For this review, take the finished solid that the model builds, in its own axes (mm). Coordinates: 2 decimals unless noted, no trailing zeros. Write each loop counter-clockwise with the first axis right and the second up, starting at its lowest first coordinate (ties: lowest second). Pieces come first, ordered by that corner, then holes. Notation, with made-up numbers: (-10.5, 54.25) -> (40.5, 54.25) arc R5 ccw to (40.5, 62.25) -> close; hole circle Ø7 at (51, 32). An arc over 180 degrees is marked (long way). One line per item, written item: value. Start each with the question number.
1) For probe 1 along Y at (x, z) = (23.55, -66.4); probe 2 along Y at (x, z) = (0, -67), list the stretches that pass through material, from the lowest coordinate up. Write a range as from..to.
2) Add section B-B (x = 15.75). State the section outline as (y, z) points, and give its area (3 significant figures).
3) Add section D-D (x = 0). State the section outline as (y, z) points.
4) Add section C-C (z = -66.8). State the section outline as (x, y) points, and give its area (3 significant figures).
5) Add section A-A (y = -23.55). State the section outline as (x, z) points, and give its area (3 significant figures).
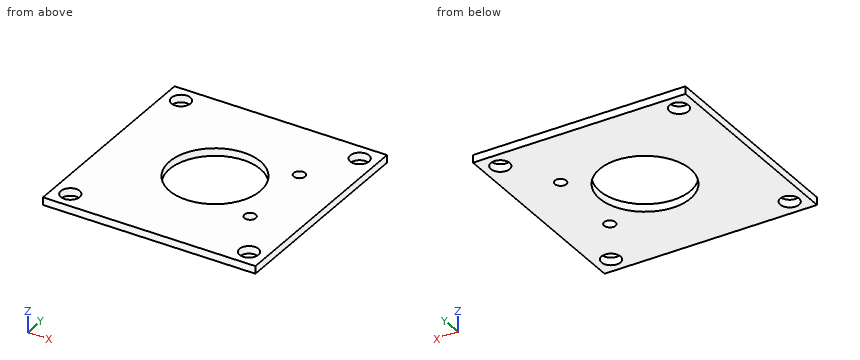
from build123d import *

# Parameters (mm, degrees)
BOX274_W                    = 56
BOX274_H                    = 56
BOX274_DEPTH                = 2
CYLINDER704_R               = 1.5
CYLINDER704_DEPTH           = 20
CYLINDER705_R               = 1.5
CYLINDER705_DEPTH           = 20
COMPOUND417_PLACEMENT_ANGLE = 90
BOX272_W                    = 20
BOX272_H                    = 8
BOX272_DEPTH                = 3
BOX271_W                    = 20
BOX271_H                    = 8
BOX271_DEPTH                = 3
BOX273_W                    = 20
BOX273_H                    = 8
BOX273_DEPTH                = 3
BOX269_W                    = 20
BOX269_H                    = 8
BOX269_DEPTH                = 3
CYLINDER697_R               = 12
CYLINDER697_DEPTH           = 20
CYLINDER702_R               = 5
CYLINDER702_DEPTH           = 4
CYLINDER689_R               = 5
CYLINDER689_DEPTH           = 4
CYLINDER693_R               = 5
CYLINDER693_DEPTH           = 4
CYLINDER698_R               = 5
CYLINDER698_DEPTH           = 4
CYLINDER699_R               = 2.5
CYLINDER699_DEPTH           = 20
CYLINDER690_R               = 2.5
CYLINDER690_DEPTH           = 20
CYLINDER694_R               = 2.5
CYLINDER694_DEPTH           = 20
CYLINDER700_R               = 2.5
CYLINDER700_DEPTH           = 20
CYLINDER696_R               = 3
CYLINDER696_DEPTH           = 5
CYLINDER696_PLACEMENT_ANGLE = 22.5
CYLINDER688_R               = 3
CYLINDER688_DEPTH           = 5
CYLINDER688_PLACEMENT_ANGLE = 67.5
CYLINDER691_R               = 3
CYLINDER691_DEPTH           = 5
CYLINDER691_PLACEMENT_ANGLE = 202.5
CYLINDER692_R               = 3
CYLINDER692_DEPTH           = 5
CYLINDER692_PLACEMENT_ANGLE = 112.5
COMPOUND416_PLACEMENT_ANGLE = 45
CYLINDER703_R               = 1.5
CYLINDER703_DEPTH           = 30
CYLINDER703_PLACEMENT_ANGLE = 22.5
CYLINDER695_R               = 1.5
CYLINDER695_DEPTH           = 30
CYLINDER695_PLACEMENT_ANGLE = 67.5
CYLINDER706_R               = 1.5
CYLINDER706_DEPTH           = 30
CYLINDER706_PLACEMENT_ANGLE = 202.5
CYLINDER701_R               = 1.5
CYLINDER701_DEPTH           = 30
CYLINDER701_PLACEMENT_ANGLE = 112.5
COMPOUND412_PLACEMENT_ANGLE = 45
BOX270_W                    = 68
BOX270_H                    = 64
BOX270_DEPTH                = 8


with BuildPart() as krychle274:
    # Box274 → Box274 (new body)
    with BuildSketch(Plane(origin=(-28, -28, -68), x_dir=(1, 0, 0), z_dir=(0, 0, 1))):
        with Locations((28, 28)):
            Rectangle(BOX274_W, BOX274_H)
    extrude(amount=BOX274_DEPTH)


with BuildPart() as obj1:
    # Cylinder704 → Cylinder704 (new body)
    with BuildSketch(Plane(origin=(15.75, 114, 59.48), x_dir=(-1, 0, 0), z_dir=(0, 1, 0))):
        Circle(CYLINDER704_R)
    extrude(amount=CYLINDER704_DEPTH)


with BuildPart() as compound417:
    # Cylinder705 → Cylinder705 (new body)
    with BuildSketch(Plane(origin=(15.75, 114, 38.52), x_dir=(-1, 0, 0), z_dir=(0, 1, 0))):
        Circle(CYLINDER705_R)
    extrude(amount=CYLINDER705_DEPTH)

    # Compound417: union obj1
    add(obj1.part)


with BuildPart() as compound417_1:
    # Compound417 placement: moved
    add(compound417.part.moved(Location((0, 49, -200))).rotate(Axis((0, 49, -200), (1, 0, 0)), COMPOUND417_PLACEMENT_ANGLE))


with BuildPart() as krychle272:
    # Box272 → Box272 (new body)
    with BuildSketch(Plane(origin=(17.55, -27.55, 31), x_dir=(1, 0, 0), z_dir=(0, 0, 1))):
        with Locations((10, 4)):
            Rectangle(BOX272_W, BOX272_H)
    extrude(amount=BOX272_DEPTH)


with BuildPart() as krychle271:
    # Box271 → Box271 (new body)
    with BuildSketch(Plane(origin=(-37.45, 19.55, 31), x_dir=(1, 0, 0), z_dir=(0, 0, 1))):
        with Locations((10, 4)):
            Rectangle(BOX271_W, BOX271_H)
    extrude(amount=BOX271_DEPTH)


with BuildPart() as krychle273:
    # Box273 → Box273 (new body)
    with BuildSketch(Plane(origin=(-37.45, -27.55, 31), x_dir=(1, 0, 0), z_dir=(0, 0, 1))):
        with Locations((10, 4)):
            Rectangle(BOX273_W, BOX273_H)
    extrude(amount=BOX273_DEPTH)


with BuildPart() as compound413:
    # Box269 → Box269 (new body)
    with BuildSketch(Plane(origin=(17.55, 19.55, 31), x_dir=(1, 0, 0), z_dir=(0, 0, 1))):
        with Locations((10, 4)):
            Rectangle(BOX269_W, BOX269_H)
    extrude(amount=BOX269_DEPTH)

    # Compound413: union Krychle272, Krychle271, Krychle273
    add(krychle272.part)
    add(krychle271.part)
    add(krychle273.part)


with BuildPart() as compound413_1:
    # Compound413 placement: moved
    add(compound413.part.moved(Location((0, 0, -4))))


with BuildPart() as obj2:
    # Cylinder697 → Cylinder697 (new body)
    with BuildSketch(Plane.XY.offset(15)):
        Circle(CYLINDER697_R)
    extrude(amount=CYLINDER697_DEPTH)


with BuildPart() as obj3:
    # Cylinder702 → Cylinder702 (new body)
    with BuildSketch(Plane(origin=(23.55, 23.55, 26), x_dir=(1, 0, 0), z_dir=(0, 0, 1))):
        Circle(CYLINDER702_R)
    extrude(amount=CYLINDER702_DEPTH)


with BuildPart() as obj4:
    # Cylinder689 → Cylinder689 (new body)
    with BuildSketch(Plane(origin=(23.55, -23.55, 26), x_dir=(1, 0, 0), z_dir=(0, 0, 1))):
        Circle(CYLINDER689_R)
    extrude(amount=CYLINDER689_DEPTH)


with BuildPart() as obj5:
    # Cylinder693 → Cylinder693 (new body)
    with BuildSketch(Plane(origin=(-23.55, 23.55, 26), x_dir=(1, 0, 0), z_dir=(0, 0, 1))):
        Circle(CYLINDER693_R)
    extrude(amount=CYLINDER693_DEPTH)


with BuildPart() as compound415:
    # Cylinder698 → Cylinder698 (new body)
    with BuildSketch(Plane(origin=(-23.55, -23.55, 26), x_dir=(1, 0, 0), z_dir=(0, 0, 1))):
        Circle(CYLINDER698_R)
    extrude(amount=CYLINDER698_DEPTH)

    # Compound415: union obj3, obj4, obj5
    add(obj3.part)
    add(obj4.part)
    add(obj5.part)


with BuildPart() as compound415_1:
    # Compound415 placement: moved
    add(compound415.part.moved(Location((0, 0, -50))))


with BuildPart() as obj6:
    # Cylinder699 → Cylinder699 (new body)
    with BuildSketch(Plane(origin=(-23.55, 23.55, 20), x_dir=(1, 0, 0), z_dir=(0, 0, 1))):
        Circle(CYLINDER699_R)
    extrude(amount=CYLINDER699_DEPTH)


with BuildPart() as obj7:
    # Cylinder690 → Cylinder690 (new body)
    with BuildSketch(Plane(origin=(-23.55, -23.55, 20), x_dir=(1, 0, 0), z_dir=(0, 0, 1))):
        Circle(CYLINDER690_R)
    extrude(amount=CYLINDER690_DEPTH)


with BuildPart() as obj8:
    # Cylinder694 → Cylinder694 (new body)
    with BuildSketch(Plane(origin=(23.55, -23.55, 20), x_dir=(1, 0, 0), z_dir=(0, 0, 1))):
        Circle(CYLINDER694_R)
    extrude(amount=CYLINDER694_DEPTH)


with BuildPart() as compound414:
    # Cylinder700 → Cylinder700 (new body)
    with BuildSketch(Plane(origin=(23.55, 23.55, 20), x_dir=(1, 0, 0), z_dir=(0, 0, 1))):
        Circle(CYLINDER700_R)
    extrude(amount=CYLINDER700_DEPTH)

    # Compound414: union obj6, obj7, obj8
    add(obj6.part)
    add(obj7.part)
    add(obj8.part)


with BuildPart() as obj9:
    # Cylinder696 → Cylinder696 (new body)
    with BuildSketch(Plane.XY):
        Circle(CYLINDER696_R)
    extrude(amount=CYLINDER696_DEPTH)


with BuildPart() as obj9_1:
    # Cylinder696 placement: moved
    add(obj9.part.moved(Location((-16, 0, 2))).rotate(Axis((-16, 0, 2), (0, 0, 1)), CYLINDER696_PLACEMENT_ANGLE))


with BuildPart() as obj10:
    # Cylinder688 → Cylinder688 (new body)
    with BuildSketch(Plane.XY):
        Circle(CYLINDER688_R)
    extrude(amount=CYLINDER688_DEPTH)


with BuildPart() as obj10_1:
    # Cylinder688 placement: moved
    add(obj10.part.moved(Location((0, 16, 2))).rotate(Axis((0, 16, 2), (0, 0, -1)), CYLINDER688_PLACEMENT_ANGLE))


with BuildPart() as obj11:
    # Cylinder691 → Cylinder691 (new body)
    with BuildSketch(Plane.XY):
        Circle(CYLINDER691_R)
    extrude(amount=CYLINDER691_DEPTH)


with BuildPart() as obj11_1:
    # Cylinder691 placement: moved
    add(obj11.part.moved(Location((16, 0, 2))).rotate(Axis((16, 0, 2), (0, 0, 1)), CYLINDER691_PLACEMENT_ANGLE))


with BuildPart() as compound416:
    # Cylinder692 → Cylinder692 (new body)
    with BuildSketch(Plane.XY):
        Circle(CYLINDER692_R)
    extrude(amount=CYLINDER692_DEPTH)


with BuildPart() as compound416_1:
    # Cylinder692 placement: moved
    add(compound416.part.moved(Location((0, -16, 2))).rotate(Axis((0, -16, 2), (0, 0, 1)), CYLINDER692_PLACEMENT_ANGLE))

    # Compound416: union obj9, obj10, obj11
    add(obj9_1.part)
    add(obj10_1.part)
    add(obj11_1.part)


with BuildPart() as compound416_2:
    # Compound416 placement: moved
    add(compound416_1.part.moved(Location((0, 0, 18))).rotate(Axis((0, 0, 18), (0, 0, 1)), COMPOUND416_PLACEMENT_ANGLE))


with BuildPart() as obj12:
    # Cylinder703 → Cylinder703 (new body)
    with BuildSketch(Plane.XY):
        Circle(CYLINDER703_R)
    extrude(amount=CYLINDER703_DEPTH)


with BuildPart() as obj12_1:
    # Cylinder703 placement: moved
    add(obj12.part.moved(Location((-16, 0, 2))).rotate(Axis((-16, 0, 2), (0, 0, 1)), CYLINDER703_PLACEMENT_ANGLE))


with BuildPart() as obj13:
    # Cylinder695 → Cylinder695 (new body)
    with BuildSketch(Plane.XY):
        Circle(CYLINDER695_R)
    extrude(amount=CYLINDER695_DEPTH)


with BuildPart() as obj13_1:
    # Cylinder695 placement: moved
    add(obj13.part.moved(Location((0, 16, 2))).rotate(Axis((0, 16, 2), (0, 0, -1)), CYLINDER695_PLACEMENT_ANGLE))


with BuildPart() as obj14:
    # Cylinder706 → Cylinder706 (new body)
    with BuildSketch(Plane.XY):
        Circle(CYLINDER706_R)
    extrude(amount=CYLINDER706_DEPTH)


with BuildPart() as obj14_1:
    # Cylinder706 placement: moved
    add(obj14.part.moved(Location((16, 0, 2))).rotate(Axis((16, 0, 2), (0, 0, 1)), CYLINDER706_PLACEMENT_ANGLE))


with BuildPart() as compound412:
    # Cylinder701 → Cylinder701 (new body)
    with BuildSketch(Plane.XY):
        Circle(CYLINDER701_R)
    extrude(amount=CYLINDER701_DEPTH)


with BuildPart() as compound412_1:
    # Cylinder701 placement: moved
    add(compound412.part.moved(Location((0, -16, 2))).rotate(Axis((0, -16, 2), (0, 0, 1)), CYLINDER701_PLACEMENT_ANGLE))

    # Compound412: union obj12, obj13, obj14
    add(obj12_1.part)
    add(obj13_1.part)
    add(obj14_1.part)


with BuildPart() as compound412_2:
    # Compound412 placement: moved
    add(compound412_1.part.moved(Location((0, 0, 50))).rotate(Axis((0, 0, 50), (0, 0, 1)), COMPOUND412_PLACEMENT_ANGLE))


with BuildPart() as common002:
    # Box270 → Box270 (new body)
    with BuildSketch(Plane(origin=(-34, -32, 26), x_dir=(1, 0, 0), z_dir=(0, 0, 1))):
        with Locations((34, 32)):
            Rectangle(BOX270_W, BOX270_H)
    extrude(amount=BOX270_DEPTH)

    # Cut275: cut Compound412
    add(compound412_2.part, mode=Mode.SUBTRACT)

    # Cut274: cut Compound416
    add(compound416_2.part, mode=Mode.SUBTRACT)

    # Cut273: cut Compound414
    add(compound414.part, mode=Mode.SUBTRACT)

    # Cut278: cut Compound415
    add(compound415_1.part, mode=Mode.SUBTRACT)

    # Cut277: cut obj2
    add(obj2.part, mode=Mode.SUBTRACT)

    # Cut276: cut Compound413
    add(compound413_1.part, mode=Mode.SUBTRACT)


with BuildPart() as common002_1:
    # Cut276 placement: moved
    add(common002.part.moved(Location((0, 0, -100))))

    # Cut279: cut Compound417
    add(compound417_1.part, mode=Mode.SUBTRACT)

    # Common002: intersect Krychle274
    add(krychle274.part, mode=Mode.INTERSECT)


solid = common002_1.part
Numbers:
1. probe 1: -28..-26.05, -21.05..21.05, 26.05..28
1. probe 2: -28..-12, 12..28
2. outline: (-28, -68) -> (-11.98, -68) -> (-11.98, -66) -> (-28, -66) -> close; (-8.98, -68) -> (8.98, -68) -> (8.98, -66) -> (-8.98, -66) -> close; (11.98, -68) -> (28, -68) -> (28, -66) -> (11.98, -66) -> close
2. area: 100 mm²
3. outline: (-28, -68) -> (-12, -68) -> (-12, -66) -> (-28, -66) -> close; (12, -68) -> (28, -68) -> (28, -66) -> (12, -66) -> close
4. outline: (-28, -28) -> (28, -28) -> (28, 28) -> (-28, 28) -> close; hole circle Ø5 at (-23.55, -23.55); hole circle Ø5 at (-23.55, 23.55); hole circle Ø24 at (0, 0); hole circle Ø3 at (15.75, -10.48); hole circle Ø3 at (15.75, 10.48); hole circle Ø5 at (23.55, -23.55); hole circle Ø5 at (23.55, 23.55)
4. area: 2,590 mm²
5. outline: (-28, -68) -> (-26.05, -68) -> (-26.05, -66) -> (-28, -66) -> close; (-21.05, -68) -> (21.05, -68) -> (21.05, -66) -> (-21.05, -66) -> close; (26.05, -68) -> (28, -68) -> (28, -66) -> (26.05, -66) -> close
5. area: 92.0 mm²
